Here's how the part is built. I have some questions about the finished solid (model axes, mm). A direction names the side the tool comes from. Round coordinates to 2 decimals unless told otherwise and drop trailing zeros. Loops run counter-clockwise (first coordinate to the right, second up) from the corner with the lowest first, then second, coordinate; pieces in that order, holes last. Notation, with made-up numbers: M -26.5,-24.5 L -3.5,-24.5 A13 cw -3.5,-3.5 Z; hole C 78,-14 d7. An arc over 180 degrees is marked long. Answer as CSV lines item,"result".
```python
from build123d import *

# Parameters (mm, degrees)
BOSS_EXTRUDE1_DEPTH = 6
CUT_EXTRUDE1_DEPTH  = 194.145023234
SKETCH5_R           = 2
CUT_EXTRUDE2_DEPTH  = 155.550962469
FILLET1_R           = 30
CHAMFER1_SIZE       = 5
FILLET2_R           = 5
SKETCH6_W           = 7
SKETCH6_H           = 10
CUT_EXTRUDE3_DEPTH  = 194.145023234
HOLE1_D             = 4.4
HOLE1_CBORE_D       = 7.5
HOLE1_CBORE_DEPTH   = 3
HOLE2_D             = 4.4
HOLE2_CBORE_D       = 7.5
HOLE2_CBORE_DEPTH   = 3
FILLET3_R           = 5
FILLET5_R           = 5
HOLE3_D             = 4.4
HOLE3_CBORE_D       = 7.5
HOLE3_CBORE_DEPTH   = 3


with BuildPart() as part:
    # Sketch1 → Boss-Extrude1 (new body)
    with BuildSketch(Plane.XY):
        Polygon((0, 0), (-138, 0), (-138, 30), (-63, 30), (-63, 40), (-138, 40), (-138, 59), (-112, 59), (-112, 87), (-90, 87), (-90, 135), (0, 135), align=None)
    extrude(amount=BOSS_EXTRUDE1_DEPTH)

    # Sketch4 → Cut-Extrude1 (cut, through all)
    with BuildSketch(Plane(origin=(0, 0, 0), x_dir=(-1, 0, 0), z_dir=(0, 0, -1))):
        Polygon((120, 40), (138, 45), (138, 40), align=None)
        Polygon((120, 30), (138, 30), (138, 25), align=None)
    extrude(amount=-CUT_EXTRUDE1_DEPTH, mode=Mode.SUBTRACT)

    # Sketch5 → Cut-Extrude2 (cut, through all)
    with BuildSketch(Plane.ZY.offset(63)):
        with Locations((3, 35)):
            Circle(SKETCH5_R)
    extrude(amount=-CUT_EXTRUDE2_DEPTH, mode=Mode.SUBTRACT)

    # Fillet1
    fillet1_edges = [part.edges().sort_by_distance(p)[0] for p in [
        (-120, 40, 3),
        (-120, 30, 3),
    ]]
    fillet(fillet1_edges, radius=FILLET1_R)

    # Chamfer1
    chamfer1_edges = [part.edges().sort_by_distance(p)[0] for p in [
        (-112, 73, 0),
        (-90, 111, 0),
    ]]
    chamfer(chamfer1_edges, length=CHAMFER1_SIZE)

    # Fillet2
    fillet2_edges = [part.edges().sort_by_distance(p)[0] for p in [
        (-138, 59, 3),
        (-138, 45, 3),
        (-138, 25, 3),
    ]]
    fillet(fillet2_edges, radius=FILLET2_R)

    # Sketch6 → Cut-Extrude3 (cut, through all)
    with BuildSketch(Plane.XY.offset(6)):
        with Locations((-3.5, 35)):
            Rectangle(SKETCH6_W, SKETCH6_H)
    extrude(amount=-CUT_EXTRUDE3_DEPTH, mode=Mode.SUBTRACT)

    # Hole1 (through all)
    with Locations(Plane.XY.offset(6)):
        with Locations((-17.4, 117), (-17.4, 80), (-17.4, 28)):
            CounterBoreHole(HOLE1_D / 2, HOLE1_CBORE_D / 2, HOLE1_CBORE_DEPTH)

    # Hole2 (through all)
    with Locations(Plane.XY.offset(6)):
        with Locations((-3, 125), (-3, 67.5), (-3, 10)):
            CounterBoreHole(HOLE2_D / 2, HOLE2_CBORE_D / 2, HOLE2_CBORE_DEPTH)

    # Fillet3
    fillet3_edges = [part.edges().sort_by_distance(p)[0] for p in [
        (-112, 59, 5.5),
        (-90, 87, 5.5),
        (-109.5, 59, 2.5),
        (-87.5, 87, 2.5),
    ]]
    fillet(fillet3_edges, radius=FILLET3_R)

    # Fillet5
    fillet5_edges = [part.edges().sort_by_distance(p)[0] for p in [
        (-109.5, 87, 2.5),
    ]]
    fillet(fillet5_edges, radius=FILLET5_R)

    # Hole3 (through all)
    with Locations(Plane.XY.offset(6)):
        with Locations((-130.844995532, 4.293591352), (-114.451398707, 7.906888356), (-87.870353785, 4.293591352)):
            CounterBoreHole(HOLE3_D / 2, HOLE3_CBORE_D / 2, HOLE3_CBORE_DEPTH)


solid = part.part
```
1. For P1, Ø8, axis at x = -130.5, y = 4.5, coming from the +Z side; P2, Ø1.5, axis at x = -97, z = 3.5, coming from the +Y side; P3, Ø2.5, axis at x = -114.45, y = 7.91, coming from the +Z side; P4, Ø2, axis at x = -18.5, y = 78.5, coming from the +Z side, each with a flat end and sliding along its axis, tell me the tip position at first contact or that it passes through.
Evaluation:
P1,"stops at z = 6"
P2,"stops at y = 87"
P3,"passes through"
P4,"stops at z = 3"
2. I want a section at C-C, the plane x = -68.5. Please give me the cut outline in (y, z).
Evaluation:
outline,"M 0,0 L 30,0 L 30,6 L 0,6 Z; M 40,0 L 135,0 L 135,6 L 40,6 Z"
3. I want a section at B-B, the plane x = -17.4. Count the separate pieces of the cut face and the enclosed holes in it, and give its area (3 significant figures).
Evaluation:
separate pieces,"4"
enclosed holes,"1"
area,"690 mm²"
4. I want a section at D-D, the plane x = -42. Please give me the cut outline in (y, z).
Evaluation:
outline,"M 0,0 L 135,0 L 135,6 L 0,6 Z; hole C 35,3 d4"
5. I want a section at A-A, the plane y = 67.5. Please give me the cut outline in (x, z).
Evaluation:
outline,"M -112,5 L -107,0 L -5.2,0 L -5.2,3 L -6.75,3 L -6.75,6 L -112,6 Z; M -0.8,0 L 0,0 L 0,3 L -0.8,3 Z"
6. Which directions (+Z, -Z, +X, -X, +Y, -Y) give clear straight access to the entire face, cutting with the end or side of a thin tool? Please do faces 1 (the flat face through (-138, 10, 3)), 2 (the flat face through (-130.9, 1.8, 3)), 3 (the flat face through (-4, 40, 3)), 4 (the flat face through (-88, 113, 3)).
Evaluation:
face 1,"+Z, -Z, -X, +Y, -Y"
face 2,"+Z"
face 3,"+Z, -Z, +X"
face 4,"-Z, -X, +Y"
7. If I drill on line 1 (Y direction, x = -3, z = 2.35); line 2 (Y direction, x = -104, z = 4.75); line 3 (Y direction, x = -86, z = 0.5), over which ranges is the centre line in solid material (lowest first)? Write a range as [from, to].
Evaluation:
line 1,"y = [0, 7.8], [12.2, 30], [40, 65.3], [69.7, 122.8], [127.2, 135]"
line 2,"y = [0, 30], [40, 87]"
line 3,"y = [0, 3.14], [5.45, 30], [40, 90.15]"
